Can you work these out from the model? Positions are in its coordinate system, mm. Coordinates: 2 decimals unless noted, no trailing zeros. Write each loop counter-clockwise with the first axis right and the second up, starting at its lowest first coordinate (ties: lowest second). Pieces come first, ordered by that corner, then holes. Notation, with made-up numbers: M 64,-34 L 83,-34 A36 cw 83,5 Z; hole C -9.75,-6 d7. An arc over 180 degrees is marked long. Answer as a JSON object with one key per item and string values. Group by question number.
from build123d import *

# Parameters (mm, degrees)
SKETCH1_W               = 76.2
SKETCH1_H               = 58.674
BOSS_EXTRUDE1_DEPTH     = 466.09
F_1_4_20_TAPPED_HOLE1_D = 5.1054


with BuildPart() as part:
    # Sketch1 → Boss-Extrude1 (new body)
    with BuildSketch(Plane(origin=(0, 0, 0), x_dir=(1, 0, 0), z_dir=(0, 1, 0))):
        with Locations((38.1, 29.337)):
            Rectangle(SKETCH1_W, SKETCH1_H)
    extrude(amount=-BOSS_EXTRUDE1_DEPTH)

    # 1/4-20 Tapped Hole1 (through all)
    with Locations(Plane(origin=(57.15, 0, -41.148), x_dir=(0, 0, 1), z_dir=(0, 1, 0))):
        with Locations((0, 0), (23.622, 0), (0, -38.1), (23.622, -38.1), (-79.662554242, -14.323198742)):
            Hole(F_1_4_20_TAPPED_HOLE1_D / 2)


solid = part.part
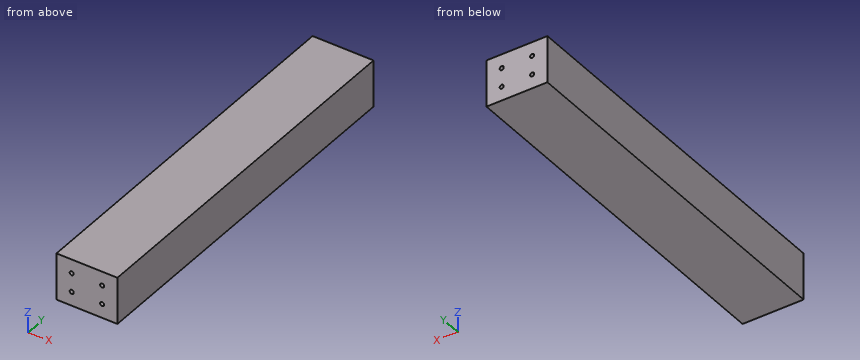
Q1. Please list where these lines run through material, in increasing order: L1, parallel to X at y = -26, z = -17.5; L2, parallel to Z at x = 57, y = -203; L3, parallel to X at y = -60, z = -19.5.
Q2. Will this pin go through, and if not, where does the flat tip stop? pin 1 (3 mm diameter, centred on x = 61, z = -32.5, fed in from +Y).
Q3. If we section it at A-A on y = -335: List the corners of the cut face in (x, z) for me.
Reply:
{
 "1": {"L1": "0 to 16.5, 21.6 to 54.6, 59.7 to 76.2", "L2": "-58.67 to -43.7, -38.6 to -20.07, -14.98 to 0", "L3": "0 to 17.43, 20.67 to 55.53, 58.77 to 76.2"},
 "2": {"pin 1": "y = 0"},
 "3": {"outline": "M 0,-58.67 L 76.2,-58.67 L 76.2,0 L 0,0 Z; hole C 19.05,-41.15 d5.11; hole C 19.05,-17.53 d5.11; hole C 57.15,-41.15 d5.11; hole C 57.15,-17.53 d5.11"}
}
